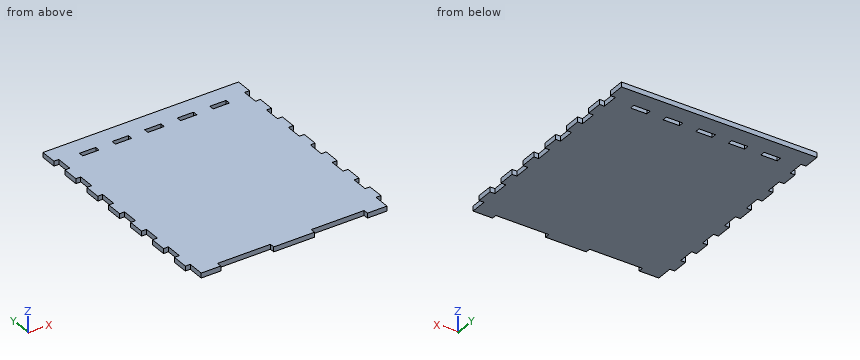
from build123d import *

# Parameters (mm, degrees)
SKETCH1_W           = 240
SKETCH1_H           = 280
BOSS_EXTRUDE1_DEPTH = 6
SKETCH3_W           = 6
SKETCH3_H           = 20
CUT_EXTRUDE1_DEPTH  = 6
SKETCH4_W           = 6
SKETCH4_H           = 20
SKETCH4_W_2         = 65
SKETCH4_H_2         = 6
CUT_EXTRUDE2_DEPTH  = 6
SKETCH5_W           = 20
SKETCH5_H           = 6
CUT_EXTRUDE3_DEPTH  = 6


with BuildPart() as part:
    # Sketch1 → Boss-Extrude1 (new body)
    with BuildSketch(Plane.XY):
        Rectangle(SKETCH1_W, SKETCH1_H)
    extrude(amount=-BOSS_EXTRUDE1_DEPTH)

    # Sketch3 → Cut-Extrude1 (cut)
    with BuildSketch(Plane.XY):
        with Locations((117, 110)):
            Rectangle(SKETCH3_W, SKETCH3_H)
        with Locations((117, 70)):
            Rectangle(SKETCH3_W, SKETCH3_H)
        with Locations((117, 30)):
            Rectangle(SKETCH3_W, SKETCH3_H)
        with Locations((117, -10)):
            Rectangle(SKETCH3_W, SKETCH3_H)
        with Locations((117, -50)):
            Rectangle(SKETCH3_W, SKETCH3_H)
        with Locations((-117, 110)):
            Rectangle(SKETCH3_W, SKETCH3_H)
        with Locations((-117, 70)):
            Rectangle(SKETCH3_W, SKETCH3_H)
        with Locations((-117, 30)):
            Rectangle(SKETCH3_W, SKETCH3_H)
        with Locations((-117, -10)):
            Rectangle(SKETCH3_W, SKETCH3_H)
        with Locations((-117, -50)):
            Rectangle(SKETCH3_W, SKETCH3_H)
        with Locations((117, -90)):
            Rectangle(SKETCH3_W, SKETCH3_H)
        with Locations((-117, -90)):
            Rectangle(SKETCH3_W, SKETCH3_H)
    extrude(amount=-CUT_EXTRUDE1_DEPTH, mode=Mode.SUBTRACT)

    # Sketch4 → Cut-Extrude2 (cut)
    with BuildSketch(Plane.XY):
        with Locations((117, -130)):
            Rectangle(SKETCH4_W, SKETCH4_H)
        with Locations((57.5, -137)):
            Rectangle(SKETCH4_W_2, SKETCH4_H_2)
        with Locations((-57.5, -137)):
            Rectangle(SKETCH4_W_2, SKETCH4_H_2)
        with Locations((-117, -130)):
            Rectangle(SKETCH4_W, SKETCH4_H)
    extrude(amount=-CUT_EXTRUDE2_DEPTH, mode=Mode.SUBTRACT)

    # Sketch5 → Cut-Extrude3 (cut)
    with BuildSketch(Plane.XY):
        with Locations((0, 115)):
            Rectangle(SKETCH5_W, SKETCH5_H)
        with Locations((-80, 115)):
            Rectangle(SKETCH5_W, SKETCH5_H)
        with Locations((40, 115)):
            Rectangle(SKETCH5_W, SKETCH5_H)
        with Locations((80, 115)):
            Rectangle(SKETCH5_W, SKETCH5_H)
        with Locations((-40, 115)):
            Rectangle(SKETCH5_W, SKETCH5_H)
    extrude(amount=-CUT_EXTRUDE3_DEPTH, mode=Mode.SUBTRACT)


solid = part.part
CAD build for the part. Positions are in the model's coordinates, mm. Round coordinates to 2 decimals unless told otherwise and drop trailing zeros. Order: outer loops, then holes, each group sorted by start corner. A loop starts at its lowest first (then second) coordinate and runs counter-clockwise, first axis right, second up. Notation, with made-up numbers: (-36.75, 88.25) - (-30.75, 88.25) arc R23 ccw to (-30.75, 115.25) - close; hole circle Ø11 at (2.5, 25.25). An arc over 180 degrees is marked (long way). Return JSON: item names as keys, results as strings.
(1) Pin check, flat tips, straight feed: pin 1 Ø3 at (y, z) = (-93, -4) entering from +X; pin 2 Ø3 at (x, z) = (-116.5, -3) entering from -Y; pin 3 Ø1.5 at (y, z) = (73.5, -3) entering from -X. Stop position of each tip, or through.
Answer key:
{"pin 1": "stops at x = 114", "pin 2": "stops at y = -120", "pin 3": "stops at x = -114"}
(2) Cut at C-C (y = -83.5). Give the cut face in (x, z), then the cut area to 3 significant figures.
Answer key:
{"outline": "(-114, -6) - (114, -6) - (114, 0) - (-114, 0) - close", "area": "1,370 mm^2"}
(3) Wall check: probe 1 along X at (y, z) = (115, -4.85); probe 2 along Y at (x, z) = (84, -1.7); probe 3 along Y at (x, z) = (0.5, -1.95). Give the ranges that are in metal, low to high. Write a range as from..to.
Answer key:
{"probe 1": "x = -114..-90, -70..-50, -30..-10, 10..30, 50..70, 90..114", "probe 2": "y = -134..112, 118..140", "probe 3": "y = -140..112, 118..140"}
(4) Cut at B-B (z = -2.75). State how many separate pieces and enclosed holes the cut face has, then the cut area to 3 significant figures.
Answer key:
{"separate pieces": "1", "enclosed holes": "5", "area": "64,100 mm^2"}
(5) Cut at A-A (x = -46.5). Give the cut face in (y, z).
Answer key:
{"outline": "(-134, -6) - (112, -6) - (112, 0) - (-134, 0) - close; (118, -6) - (140, -6) - (140, 0) - (118, 0) - close"}
